Work out the finished part from the listing and answer in its coordinate system (mm). Coordinates: 2 decimals unless noted, no trailing zeros. Order: outer loops, then holes, each group sorted by start corner. A loop starts at its lowest first (then second) coordinate and runs counter-clockwise, first axis right, second up. Notation, with made-up numbers: (22, 70.5) -> (27, 70.5) arc R34 ccw to (27, 108.5) -> close; hole circle Ø4 at (-8.5, 43.25). An arc over 180 degrees is marked (long way). Use one line per item in the form item = value.
from build123d import *

# Parameters (mm, degrees)
SKETCH1_W           = 50.8
SKETCH1_H           = 101.6
BOSS_EXTRUDE1_DEPTH = 76.2
CHAMFER1_SIZE       = 12.7
CHAMFER1_SIZE2      = 50.8
CHAMFER2_SIZE       = 12.7
CHAMFER2_SIZE2      = 50.8
CHAMFER3_SIZE       = 12.7
CHAMFER3_SIZE2      = 50.8
CHAMFER4_SIZE       = 12.7
CHAMFER4_SIZE2      = 50.8


with BuildPart() as part:
    # Sketch1 → Boss-Extrude1 (new body)
    with BuildSketch(Plane(origin=(0, 0, 0), x_dir=(1, 0, 0), z_dir=(0, 1, 0))):
        Rectangle(SKETCH1_W, SKETCH1_H)
    extrude(amount=BOSS_EXTRUDE1_DEPTH)

    # Chamfer1
    chamfer1_edges = [part.edges().sort_by_distance(p)[0] for p in [
        (25.4, 0, 0),
    ]]
    chamfer1_side = [part.faces().sort_by_distance(p)[0] for p in [
        (0, 0, 0),
    ]]
    chamfer(chamfer1_edges, length=CHAMFER1_SIZE, length2=CHAMFER1_SIZE2, reference=chamfer1_side[0])

    # Chamfer2
    chamfer2_edges = [part.edges().sort_by_distance(p)[0] for p in [
        (-25.4, 0, 0),
    ]]
    chamfer2_side = [part.faces().sort_by_distance(p)[0] for p in [
        (-6.35, 0, 0),
    ]]
    chamfer(chamfer2_edges, length=CHAMFER2_SIZE, length2=CHAMFER2_SIZE2, reference=chamfer2_side[0])

    # Chamfer3
    chamfer3_edges = [part.edges().sort_by_distance(p)[0] for p in [
        (0, 0, 50.8),
    ]]
    chamfer3_side = [part.faces().sort_by_distance(p)[0] for p in [
        (0, 0, 0),
    ]]
    chamfer(chamfer3_edges, length=CHAMFER3_SIZE, length2=CHAMFER3_SIZE2, reference=chamfer3_side[0])

    # Chamfer4
    chamfer4_edges = [part.edges().sort_by_distance(p)[0] for p in [
        (0, 0, -50.8),
    ]]
    chamfer4_side = [part.faces().sort_by_distance(p)[0] for p in [
        (0, 0, -6.35),
    ]]
    chamfer(chamfer4_edges, length=CHAMFER4_SIZE, length2=CHAMFER4_SIZE2, reference=chamfer4_side[0])


solid = part.part
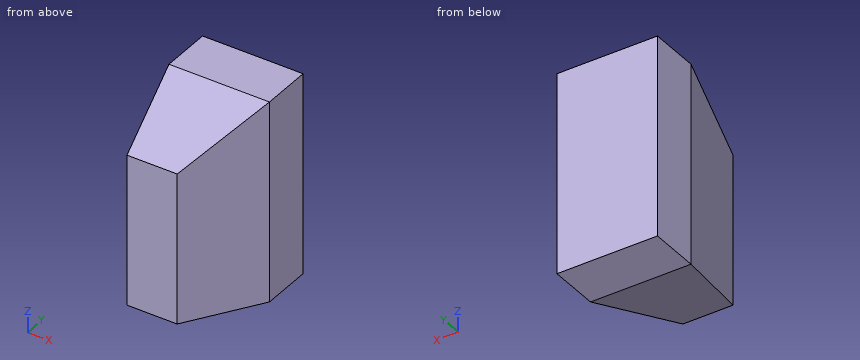
(1) Each of these flat-tipped pins is pushed along its axis until it touches: P1, Ø10, axis at x = 1.5, y = 42.5, coming from the +Z side (3 decimals); P2, Ø4, axis at x = 8.5, y = 19.5, coming from the -Z side (3 decimals); P3, Ø4, axis at y = 28, z = -37.5, coming from the +X side. Where does it stop, or does it pass through?
Data:
P1 = 49.975
P2 = -43.475
P3 = 20.2
(2) Straight lines are drawn through the part: line 1 along Z through (x, y) = (7, 29); line 2 along Z through (x, y) = (2, 37); line 3 along X through (y, z) = (11, -11). For each, find the intervals that lie inside material, in ascending order.
Data:
line_1 = -45.35 to 45.35
line_2 = -47.35 to 47.35
line_3 = -15.45 to 15.45
(3) Section A-A on x = 9.5 is taken. Write down the section's boundary in (y, z).
Data:
outline = (0, -38.1) -> (50.8, -50.8) -> (76.2, -50.8) -> (76.2, 50.8) -> (50.8, 50.8) -> (0, 38.1) -> close
(4) Section B-B on y = 28 is taken. Write down the section's boundary in (x, z), plus the area to 3 significant figures.
Data:
outline = (-19.7, -45.1) -> (19.7, -45.1) -> (19.7, 45.1) -> (-19.7, 45.1) -> close
area = 3,550 mm²
(5) Section D-D on y = 37 is taken. Write down the section's boundary in (x, z).
Data:
outline = (-21.95, -47.35) -> (21.95, -47.35) -> (21.95, 47.35) -> (-21.95, 47.35) -> close
(6) Section C-C on z = 22.5 is taken. Write down the section's boundary in (x, y), plus the area to 3 significant figures.
Data:
outline = (-25.4, 50.8) -> (-12.7, 0) -> (12.7, 0) -> (25.4, 50.8) -> (25.4, 76.2) -> (-25.4, 76.2) -> close
area = 3,230 mm²
